Job drawing, mm, ordinate dimensions from the low corner. One solid piece. A direction names the side the tool comes from. Coordinates: 2 decimals unless noted, no trailing zeros. Write each loop counter-clockwise with the first axis right and the second up, starting at its lowest first coordinate (ties: lowest second). Pieces come first, ordered by that corner, then holes. Notation, with made-up numbers: (83, 18) - (142, 18) arc R24 ccw to (142, 38) - close; hole circle Ø6 at (-10.5, 85). An arc over 180 degrees is marked (long way). Use a Markdown table: item, result.
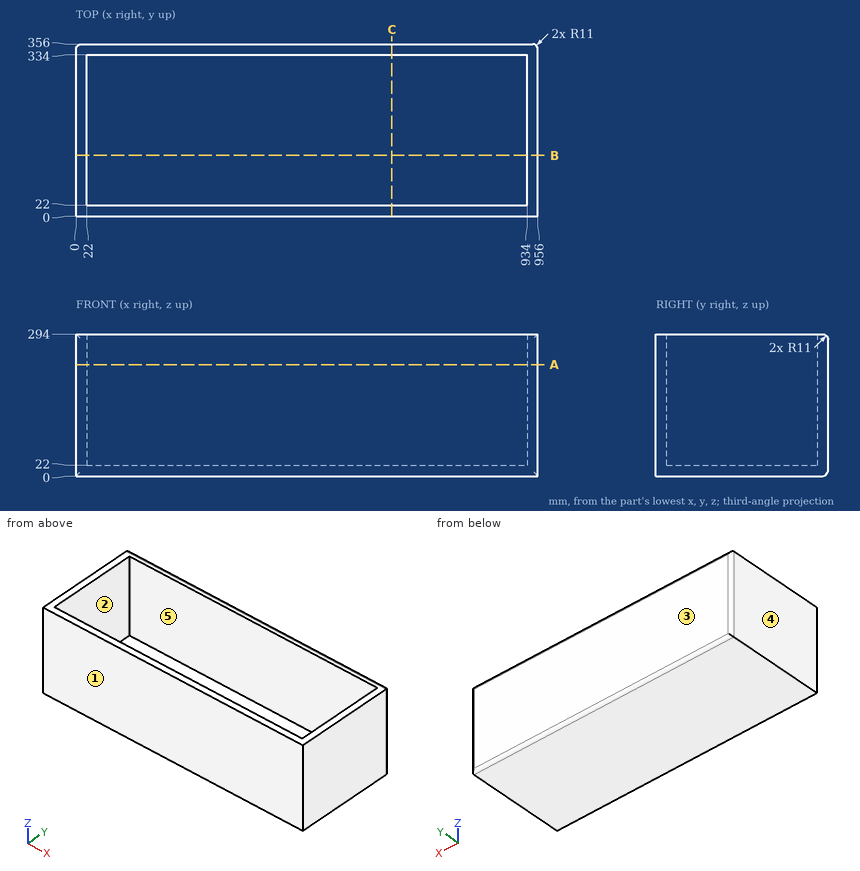
Item 1: Band-saw the part on A-A, the plane z = 230.5. Give the cut face in (x, y), then the cut area to 3 significant figures.
From the geometry:
| item | result |
|---|---|
| outline | (0, 0) - (956, 0) - (956, 345) arc R11 ccw to (945, 356) - (11, 356) arc R11 ccw to (0, 345) - close; hole (22, 22) - (934, 22) - (934, 334) - (22, 334) - close |
| area | 55,700 mm^2 |
Item 2: Drop a flat-ended pin along its axis: P1, Ø1, axis at x = 558, y = 275.5, coming from the +Z side. Give the stop position or say it passes through.
From the geometry:
| item | result |
|---|---|
| P1 | z = 22 |
Item 3: Which spindle directions (+Z, -Z, +X, -X, +Y, -Y) get a long thin tool onto all of the face, cutting with end or side? Do the marked faces 1 and 2. Say none if no direction does.
From the geometry:
| item | result |
|---|---|
| face 1 | +Z, -Z, +X, -X, -Y |
| face 2 | +Z |
Item 4: Band-saw the part on C-C, the plane x = 653.5. Give the cut face in (y, z).
From the geometry:
| item | result |
|---|---|
| outline | (0, 0) - (345, 0) arc R11 ccw to (356, 11) - (356, 283) arc R11 ccw to (345, 294) - (334, 294) - (334, 22) - (22, 22) - (22, 294) - (0, 294) - close |
Item 5: Band-saw the part on B-B, the plane y = 125.5. Give the cut face in (x, z), then the cut area to 3 significant figures.
From the geometry:
| item | result |
|---|---|
| outline | (0, 0) - (956, 0) - (956, 294) - (934, 294) - (934, 22) - (22, 22) - (22, 294) - (0, 294) - close |
| area | 33,000 mm^2 |
Item 6: Two-plate mould, pull along X, no slides. Class the marked faces 3, 4 and 5: pulls with the +X half, pulls with the -X half, needs draft (parallel to the pull), parting line crosses it, or undercut.
From the geometry:
| item | result |
|---|---|
| face 3 | needs draft |
| face 4 | pulls with the -X half |
| face 5 | undercut |
Item 7: Drill centre lines: probe 1 along X at (y, z) = (213, 266.5); probe 2 along Y at (x, z) = (787.5, 148.5); probe 3 along Z at (x, y) = (128, 209.5). Where is each one in solid material? Low to high.
From the geometry:
| item | result |
|---|---|
| probe 1 | 0 to 22, 934 to 956 |
| probe 2 | 0 to 22, 334 to 356 |
| probe 3 | 0 to 22 |
